Design review of the part built by this model. Coordinates are the model's own, in mm. Give positions to 0.01 mm unless a question says otherwise; leave off trailing zeros. Loops run counter-clockwise (first coordinate to the right, second up) from the corner with the lowest first, then second, coordinate; pieces in that order, holes last. Notation, with made-up numbers: (-27.5, 8) - (-20.5, 8) arc R24 cw to (-20.5, 25) - close; hole circle Ø4 at (48.25, 17). An arc over 180 degrees is marked (long way). Write each question's results on one line, items separated by ' | '.
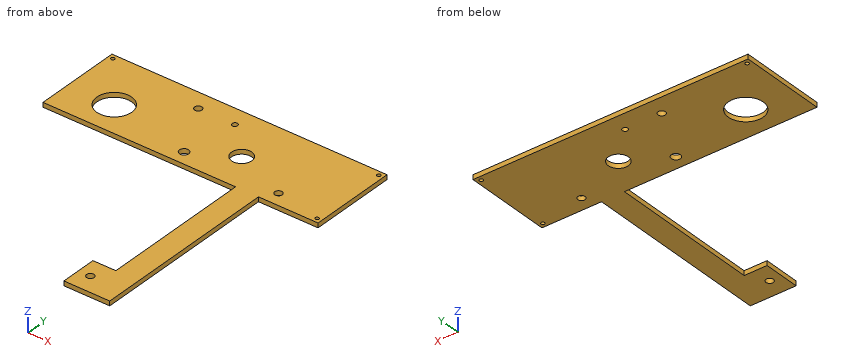
```python
from build123d import *

# Parameters (mm, degrees)
SKETCH1_R      = 4
SKETCH1_R_2    = 11
SKETCH1_R_3    = 19
SKETCH1_R_4    = 5
SKETCH1_R_5    = 3
SKETCH1_R_6    = 2
EXTRUDE1_DEPTH = 5


with BuildPart() as part:
    # Sketch1 → Extrude1 (new body)
    with BuildSketch(Plane.XY):
        Polygon((105.426271186, -213.287288136), (55.426271186, -213.287288136), (55.426271186, -173.287288136), (80.426271186, -173.287288136), (80.426271186, -8.287288136), (-129.573728814, -8.287288136), (-129.573728814, 86.712711864), (170.426271186, 86.712711864), (170.426271186, -8.287288136), (105.426271186, -8.287288136), align=None)
        with Locations((68.426271186, -193.287288136)):
            Circle(SKETCH1_R, mode=Mode.SUBTRACT)
        with Locations((115.426271186, 6.712711864)):
            Circle(SKETCH1_R, mode=Mode.SUBTRACT)
        with Locations((55.426271186, 31.712711864)):
            Circle(SKETCH1_R_2, mode=Mode.SUBTRACT)
        with Locations((-79.573728814, 26.712711864)):
            Circle(SKETCH1_R_3, mode=Mode.SUBTRACT)
        with Locations((12.426271186, 6.712711864)):
            Circle(SKETCH1_R_4, mode=Mode.SUBTRACT)
        with Locations((20.426271186, 66.712711864)):
            Circle(SKETCH1_R_5, mode=Mode.SUBTRACT)
        with Locations((-124.573728814, 81.712711864)):
            Circle(SKETCH1_R_6, mode=Mode.SUBTRACT)
        with Locations((165.426271186, 81.712711864)):
            Circle(SKETCH1_R_6, mode=Mode.SUBTRACT)
        with Locations((165.426271186, -3.287288136)):
            Circle(SKETCH1_R_6, mode=Mode.SUBTRACT)
        with Locations((-19.573728814, 66.712711864)):
            Circle(SKETCH1_R, mode=Mode.SUBTRACT)
    extrude(amount=EXTRUDE1_DEPTH)


solid = part.part
```
Item 1: We need section D-D on x = 146.5. Give the boundary of the cut face in (y, z), then the cut area to 3 significant figures.
Output values:
outline: (-8.29, 0) - (86.71, 0) - (86.71, 5) - (-8.29, 5) - close | area: 475 mm²
Item 2: We need section A-A on x = 12.5. Give the boundary of the cut face in (y, z).
Output values:
outline: (-8.29, 0) - (1.71, 0) - (1.71, 5) - (-8.29, 5) - close; (11.71, 0) - (86.71, 0) - (86.71, 5) - (11.71, 5) - close
Item 3: We need section C-C on y = -177. Give the boundary of the cut face in (x, z), then the cut area to 3 significant figures.
Output values:
outline: (55.43, 0) - (105.43, 0) - (105.43, 5) - (55.43, 5) - close | area: 250 mm²
Item 4: Wall thickness on probe 1 along X at (y, z) = (67, 1.1); probe 2 along X at (y, z) = (6, 1.35); probe 3 along Y at (x, z) = (58, 1.15): over which ranges is each line inside the solid? List them lowest first.
Output values:
probe 1: x = -129.57 to -23.56, -15.58 to 17.44, 23.41 to 170.43 | probe 2: x = -129.57 to 7.48, 17.38 to 111.49, 119.36 to 170.43 | probe 3: y = -213.29 to -173.29, -8.29 to 21.02, 42.41 to 86.71
Item 5: Clearance check with flat-ended pins moving along their axes: P1, Ø2.5, axis at y = -74.5, z = 1.5, coming from the -X side; P2, Ø8, axis at x = 20.43, y = 66.71, coming from the -Z side; P3, Ø1.5, axis at y = -144.5, z = 3, coming from the +X side; P4, Ø1.5, axis at x = 11, z = 2, coming from the -Y side. State where each tip first meets the part, or that it passes through.
Output values:
P1: stops at x = 80.43 | P2: stops at z = 0 | P3: stops at x = 105.43 | P4: stops at y = -8.29
Item 6: We need section B-B on z = 3.85. Give the number of separate pieces and of enclosed holes in the cut face, then the cut area to 3 significant figures.
Output values:
separate pieces: 1 | enclosed holes: 10 | area: 32,800 mm²
